The listing builds one solid part. Answer for the finished solid, in the listing's coordinates (mm). Coordinates: 2 decimals unless noted, no trailing zeros. Order: outer loops, then holes, each group sorted by start corner. A loop starts at its lowest first (then second) coordinate and runs counter-clockwise, first axis right, second up. Notation, with made-up numbers: (-32.5, 66.5) - (-13.5, 66.5) arc R28 ccw to (-13.5, 88.5) - close; hole circle Ø10 at (-10.5, 33). An arc over 180 degrees is marked (long way). Use a Markdown table: item, result. Add a question column.
Item 1: The part is cut by section C-C, the plane x = 114. Give the vertices of the cut face in (y, z), then the cut area to 3 significant figures.
Item 2: Flat-ended cylindrical pins translate along their axes: P1, Ø2, axis at y = 50.5, z = -4.5, coming from the -X side; P2, Ø2, axis at x = 39.5, z = -2.5, coming from the -Y side; P3, Ø2, axis at y = 40, z = -4, coming from the -X side. Find the tip coordinate at first contact, or state that the pin passes through.
Item 3: Find the intervals of material crossed by line 1 along Y through (x, z) = (-33, -1.5); line 2 along Y through (x, z) = (88.5, 3.25); line 3 along X through (y, z) = (70.5, -0.5), in increasing order.
Item 4: The part is cut by section A-A, the plane z = -1. Give the vertices of the cut face in (x, y), then the cut area to 3 significant figures.
Item 5: The part is cut by section B-B, the plane y = 35.5. Give the vertices of the cut face in (x, z), then the cut area to 3 significant figures.
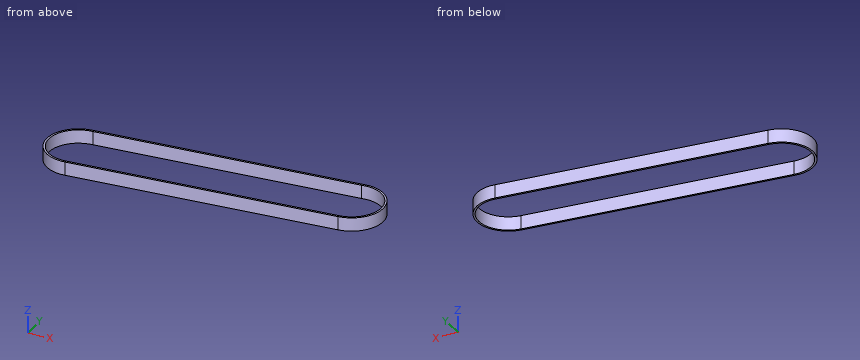
from build123d import *

# Parameters (mm, degrees)
Y_KSEKLIK_EKSTR_ZYON1_DEPTH = 7.5


with BuildPart() as part:
    # Çizim1 → Yükseklik-Ekstrüzyon1 (new body, symmetric)
    with BuildSketch(Plane(origin=(0, 0, 0), x_dir=(-1, 0, 0), z_dir=(0, 0, 1))):
        with BuildLine():
            Line((72.328772259, -16.644229091), (-218.671227741, -43.144229091))
            ThreePointArc((-218.671227741, -43.144229091), (-250.352847691, -81.174150959), (-212.322925823, -112.855770909))
            Line((-212.322925823, -112.855770909), (78.677074177, -86.355770909))
            ThreePointArc((78.677074177, -86.355770909), (110.358694128, -48.325849041), (72.328772259, -16.644229091))
        make_face()
        with BuildLine():
            ThreePointArc((-209.8089095, -110.3633999), (-248.069420133, -82.334437532), (-218.470252737, -45.27531322))
            Line((-218.470252737, -45.27531322), (72.535281972, -18.836231788))
            ThreePointArc((72.535281972, -18.836231788), (108.250828228, -49.682483602), (76.168067869, -84.291557312))
            Line((76.168067869, -84.291557312), (-209.8089095, -110.3633999))
        make_face(mode=Mode.SUBTRACT)
    extrude(amount=Y_KSEKLIK_EKSTR_ZYON1_DEPTH, both=True)


solid = part.part
Solution:
| question | item | result |
|---|---|---|
| 1 | outline | (33.61, -7.5) - (35.78, -7.5) - (35.78, 7.5) - (33.61, 7.5) - close; (101.63, -7.5) - (103.9, -7.5) - (103.9, 7.5) - (101.63, 7.5) - close |
| 1 | area | 66.7 mm2 |
| 2 | P1 | stops at x = -110.5 |
| 2 | P2 | stops at y = 26.74 |
| 2 | P3 | stops at x = -108.89 |
| 3 | line 1 | y = 20.23 to 22.43, 88.23 to 90.52 |
| 3 | line 2 | y = 31.29 to 33.47, 99.3 to 101.58 |
| 3 | line 3 | x = -104.9 to -102.24, 247.49 to 249.68 |
| 4 | outline | (-78.68, 86.36) arc R35 ccw to (-72.33, 16.64) - (218.67, 43.14) arc R35 ccw to (212.32, 112.86) - close; hole (-76.17, 84.29) arc R32.8 ccw (long way) to (-72.54, 18.84) - (218.47, 45.28) arc R32.86 ccw (long way) to (209.81, 110.36) - close |
| 4 | area | 1,760 mm2 |
| 5 | outline | (-106.63, -7.5) - (-104.13, -7.5) - (-104.13, 7.5) - (-106.63, 7.5) - close; (110.88, -7.5) - (134.73, -7.5) - (134.73, 7.5) - (110.88, 7.5) - close |
| 5 | area | 395 mm2 |
